Can you work these out from the drawing? Everything is in mm from the part's minimum corner. Round coordinates to 2 decimals unless told otherwise and drop trailing zeros. Loops run counter-clockwise (first coordinate to the right, second up) from the corner with the lowest first, then second, coordinate; pieces in that order, holes last. Notation, with made-up numbers: M 30,-15.75 L 43,-15.75 A20 ccw 43,11.25 Z; hole C -18.75,-32 d1. An arc over 180 degrees is marked long. Use a Markdown table: item, result.
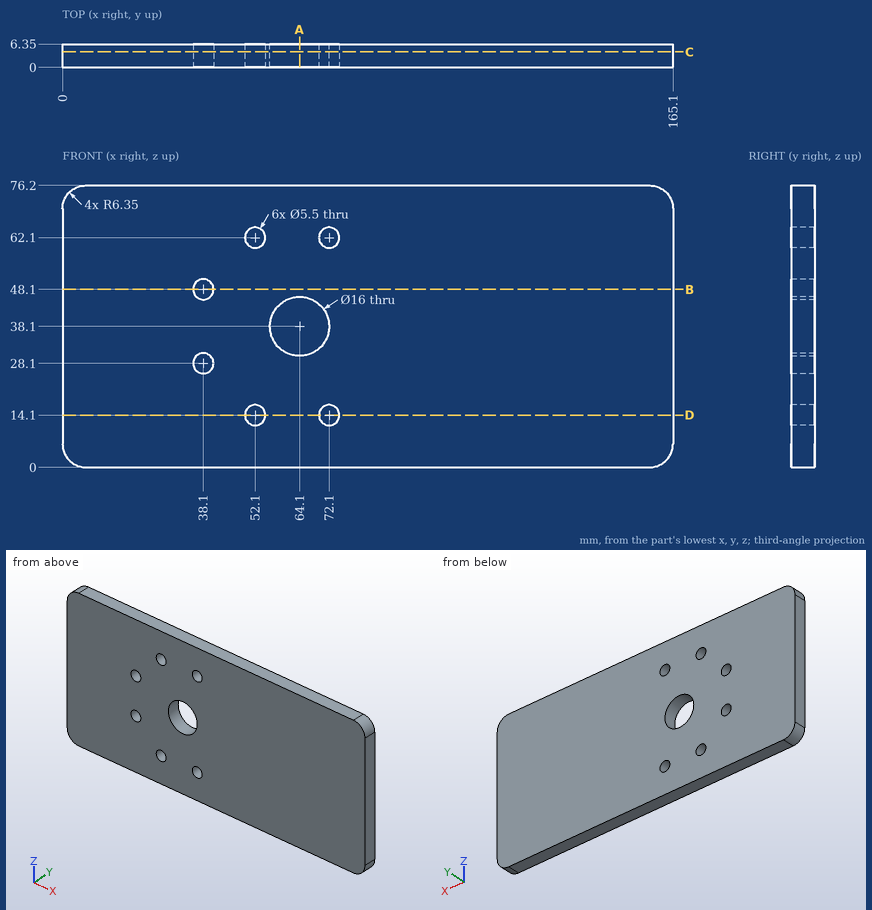
Q1. Imagine slicing it at A-A, the plane x = 64.1. Please give me the cut outline in (y, z).
Return value:
| item | result |
|---|---|
| outline | M 0,0 L 6.35,0 L 6.35,30.1 L 0,30.1 Z; M 0,46.1 L 6.35,46.1 L 6.35,76.2 L 0,76.2 Z |
Q2. I need wall thicknesses on line 1 (Z direction, x = 52.1, y = 1.5); line 2 (X direction, y = 2.25, z = 38.1); line 3 (X direction, y = 4.5, z = 28.1). Which ranges of each line are inside material? Lowest first, please. Write a range as from..to.
Return value:
| item | result |
|---|---|
| line 1 | z = 0..11.35, 16.85..59.35, 64.85..76.2 |
| line 2 | x = 0..56.1, 72.1..165.1 |
| line 3 | x = 0..35.35, 40.85..165.1 |
Q3. Imagine slicing it at C-C, the plane y = 4.25. Please give me the cut outline in (x, z), then the cut area to 3 significant figures.
Return value:
| item | result |
|---|---|
| outline | M 0,6.35 A6.35 ccw 6.35,0 L 158.75,0 A6.35 ccw 165.1,6.35 L 165.1,69.85 A6.35 ccw 158.75,76.2 L 6.35,76.2 A6.35 ccw 0,69.85 Z; hole C 38.1,28.1 d5.5; hole C 38.1,48.1 d5.5; hole C 52.1,14.1 d5.5; hole C 52.1,62.1 d5.5; hole C 64.1,38.1 d16; hole C 72.1,14.1 d5.5; hole C 72.1,62.1 d5.5 |
| area | 12,200 mm^2 |
Q4. Will this pin go through, and if not, where does the flat tip stop? P1, Ø1, axis at x = 40, z = 11.5, coming from the -Y side.
Return value:
| item | result |
|---|---|
| P1 | stops at y = 0 |
Q5. Imagine slicing it at B-B, the plane z = 48.1. Please give me the cut outline in (x, y).
Return value:
| item | result |
|---|---|
| outline | M 0,0 L 35.35,0 L 35.35,6.35 L 0,6.35 Z; M 40.85,0 L 165.1,0 L 165.1,6.35 L 40.85,6.35 Z |
Q6. Imagine slicing it at D-D, the plane z = 14.1. Please give me the cut outline in (x, y).
Return value:
| item | result |
|---|---|
| outline | M 0,0 L 49.35,0 L 49.35,6.35 L 0,6.35 Z; M 54.85,0 L 69.35,0 L 69.35,6.35 L 54.85,6.35 Z; M 74.85,0 L 165.1,0 L 165.1,6.35 L 74.85,6.35 Z |
